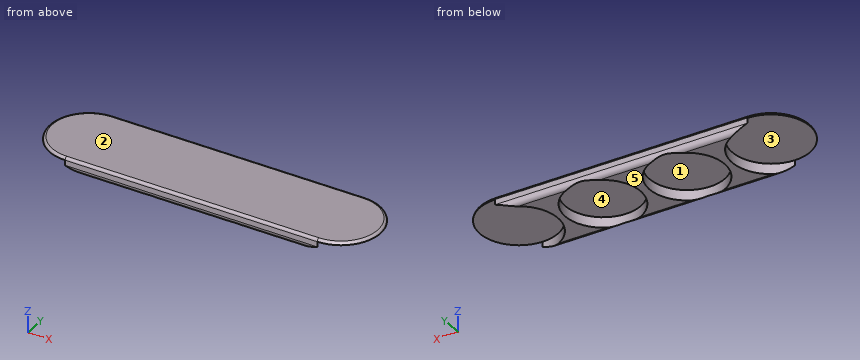
```python
from build123d import *

# Parameters (mm, degrees)
F0_R        = 14.5
F1_DEPTH    = 5
F2_DEPTH    = 4
F3_T1_DEPTH = 113
F4_R        = 0.99999


# Not quite as in the source:
# - a fillet or chamfer that OpenCascade refuses, or shapes differently, is made with other operations: its cross-section is extruded or revolved along the edge and cut away or added
# - a fillet or chamfer is up to 0.001 mm smaller than in the source, because OpenCascade refuses the exact size


with BuildPart() as f1:
    # F0 (on Top) → F1 (new body)
    with BuildSketch(Plane.XY):
        with BuildLine():
            ThreePointArc((47, 0), (42.6066017178, 10.6066017178), (32, 15))
            ThreePointArc((32, 15), (17, 0), (32, -15))
            ThreePointArc((32, -15), (42.6066017178, -10.6066017178), (47, 0))
        make_face()
        with BuildLine():
            ThreePointArc((-64, 15), (-53.3933982822, 10.6066017178), (-49, 0))
            ThreePointArc((-49, 0), (-53.3933982822, -10.6066017178), (-64, -15))
            Line((-64, -15), (32, -15))
            ThreePointArc((32, -15), (17, 0), (32, 15))
            Line((32, 15), (-64, 15))
        make_face()
        with Locations((-32, 0)):
            Circle(F0_R, mode=Mode.SUBTRACT)
        Circle(F0_R, mode=Mode.SUBTRACT)
        Circle(F0_R)
        with Locations((-32, 0)):
            Circle(F0_R)
        with BuildLine():
            ThreePointArc((-64, -15), (-53.3933982822, -10.6066017178), (-49, 0))
            ThreePointArc((-49, 0), (-53.3933982822, 10.6066017178), (-64, 15))
            ThreePointArc((-64, 15), (-79, 0), (-64, -15))
        make_face()
    extrude(amount=F1_DEPTH)

    # F0 (on Top) → F2 (cut)
    with BuildSketch(Plane.XY):
        with BuildLine():
            ThreePointArc((47, 0), (42.6066017178, 10.6066017178), (32, 15))
            ThreePointArc((32, 15), (17, 0), (32, -15))
            ThreePointArc((32, -15), (42.6066017178, -10.6066017178), (47, 0))
        make_face()
        Circle(F0_R)
        with Locations((-32, 0)):
            Circle(F0_R)
        with BuildLine():
            ThreePointArc((-64, -15), (-53.3933982822, -10.6066017178), (-49, 0))
            ThreePointArc((-49, 0), (-53.3933982822, 10.6066017178), (-64, 15))
            ThreePointArc((-64, 15), (-79, 0), (-64, -15))
        make_face()
    extrude(amount=F2_DEPTH, mode=Mode.SUBTRACT)

    # F3: fillet of radius 2 on 2 edges, made by hand

    # F3_s2 → F3_t1 (cut)
    with BuildSketch(Plane.YZ.offset(-72.5)):
        with BuildLine():
            ThreePointArc((-13, 0), (-14.4142135624, 0.5857864376), (-15, 2))
            Line((-15, 2), (-15, 0))
            Line((-15, 0), (-13, 0))
        make_face()
        with BuildLine():
            ThreePointArc((15, 2), (14.4142135624, 0.5857864376), (13, 0))
            Line((13, 0), (15, 0))
            Line((15, 0), (15, 2))
        make_face()
    extrude(amount=F3_T1_DEPTH, mode=Mode.SUBTRACT)

    # F4 (radius 1 in the source; OpenCascade refuses exactly that, so slightly less here)
    f4_edges = [f1.edges().sort_by_distance(p)[0] for p in [
        (47, 0, 5),
        (-16, 15, 5),
        (-79, 0, 5),
        (-16, -15, 5),
    ]]
    fillet(f4_edges, radius=F4_R)


solid = f1.part
```
The listing builds one solid part. Answer for the finished solid, in the listing's coordinates (mm). Face numbers are marked on the shaded views. A direction names the side the tool comes from. Coordinates: 2 decimals unless noted, no trailing zeros. Write each loop counter-clockwise with the first axis right and the second up, starting at its lowest first coordinate (ties: lowest second). Pieces come first, ordered by that corner, then holes. Notation, with made-up numbers: (-17.5, 50.5) - (10.5, 50.5) arc R29 ccw to (10.5, 74.5) - close; hole circle Ø4 at (7, 43.25). An arc over 180 degrees is marked (long way). One line per item, written item: value.
1) Consider line 1 along X through (y, z) = (0, 1.8); line 2 along X through (y, z) = (10, 3.85); line 3 along Y through (x, z) = (0, 2.5). Determine where each line is inside the solid, lowest interval first. Write a range as from..to.
Geometry check:
line 1: x = -49..-46.5, -17.5..-14.5, 14.5..17
line 2: x = -52.82..-42.5, -21.5..-10.5, 10.5..20.82
line 3: y = -15..-14.5, 14.5..15
2) For a pull along Y with two mould halves and no side action, classify the marked faces 1 and 2 as pulls with the +Y half, pulls with the -Y half, needs draft (parallel to the pull), parting line crosses it, or undercut.
Geometry check:
face 1: undercut
face 2: needs draft
3) A tool of negligible diameter and unlimited length cuts with its end or side. For the marked faces 3, 4 and 5, from which of +Z, -Z, +X, -X, +Y, -Y can it reach the whole face along a straight path? Write none if from no direction.
Geometry check:
face 3: -Z, -X
face 4: -Z
face 5: -Z, +X, -X, +Y, -Y
4) Find section B-B (x = -22). Give the vertices of the cut face in (y, z), and give its area (3 significant figures).
Geometry check:
outline: (-15, 2) arc R2 ccw to (-13, 0) - (-10.5, 0) - (-10.5, 4) - (10.5, 4) - (10.5, 0) - (13, 0) arc R2 ccw to (15, 2) - (15, 4) arc R1 ccw to (14, 5) - (-14, 5) arc R1 ccw to (-15, 4) - close
area: 63.9 mm2
5) This flat-tipped pin is pushed along its axis until it touches: pin 1 Ø4 at (x, y) = (-24.5, 0) entering from -Z. Where does it stop, or does it pass through?
Geometry check:
pin 1: stops at z = 4
6) Find section A-A (z = 2.8). Give the vertices of the cut face in (x, y), and give its area (3 significant figures).
Geometry check:
outline: (-64, -15) - (32, -15) arc R15 cw to (32, 15) - (-64, 15) arc R15 cw to start; hole circle Ø29 at (-32, 0); hole circle Ø29 at (0, 0)
area: 852 mm2
7) Find section C-C (x = -59). Give the vertices of the cut face in (y, z), and give its area (3 significant figures).
Geometry check:
outline: (-15, 2) arc R2 ccw to (-14.14, 0.36) - (-14.14, 4) - (14.14, 4) - (14.14, 0.36) arc R2 ccw to (15, 2) - (15, 4) arc R1 ccw to (14, 5) - (-14, 5) arc R1 ccw to (-15, 4) - close
area: 35.0 mm2
